```python
from build123d import *

# Parameters (mm, degrees)
F0_R     = 1.5
F1_DEPTH = 11
F2_W     = 61
F2_H     = 1
F2_H_2   = 18
F3_DEPTH = 15
F4_DEPTH = 1
F5_DEPTH = 10.5


with BuildPart() as f1:
    # F0 (on Top) → F1 (new body, symmetric)
    with BuildSketch(Plane.XY):
        Polygon((-4.5, 30.5), (-15, 30.5), (-15, -30.5), (-4.5, -30.5), (4.5, -30.5), (15, -30.5), (15, 30.5), (4.5, 30.5), align=None)
        with Locations((-5.5, -27.5)):
            Circle(F0_R, mode=Mode.SUBTRACT)
        with Locations((5.5, -27.5)):
            Circle(F0_R, mode=Mode.SUBTRACT)
        with Locations((-5.5, 27.5)):
            Circle(F0_R, mode=Mode.SUBTRACT)
        with Locations((5.5, 27.5)):
            Circle(F0_R, mode=Mode.SUBTRACT)
        with Locations((5.5, -27.5)):
            Circle(F0_R)
        with Locations((-5.5, -27.5)):
            Circle(F0_R)
        with Locations((-5.5, 27.5)):
            Circle(F0_R)
        with Locations((5.5, 27.5)):
            Circle(F0_R)
        Polygon((-3.5, 31.5), (-4.5, 30.5), (4.5, 30.5), (3.5, 31.5), align=None)
        Polygon((4.5, -30.5), (-4.5, -30.5), (-3.5, -31.5), (3.5, -31.5), align=None)
    extrude(amount=F1_DEPTH, both=True)

    # F2 (on Right) → F3 (cut, symmetric)
    with BuildSketch(Plane.YZ):
        with Locations((0, 9.5)):
            Rectangle(F2_W, F2_H)
        Rectangle(F2_W, F2_H_2)
        with Locations((0, -9.5)):
            Rectangle(F2_W, F2_H)
    extrude(amount=F3_DEPTH, both=True, mode=Mode.SUBTRACT)

    # F2 (on Right) → F4 (join, symmetric)
    with BuildSketch(Plane.YZ):
        with Locations((0, 9.5)):
            Rectangle(F2_W, F2_H)
        Rectangle(F2_W, F2_H_2)
        with Locations((0, -9.5)):
            Rectangle(F2_W, F2_H)
    extrude(amount=F4_DEPTH, both=True)

    # F0 (on Top) → F5 (cut, symmetric)
    with BuildSketch(Plane.XY):
        with Locations((-5.5, -27.5)):
            Circle(F0_R)
        with Locations((5.5, -27.5)):
            Circle(F0_R)
        with Locations((5.5, 27.5)):
            Circle(F0_R)
        with Locations((-5.5, 27.5)):
            Circle(F0_R)
    extrude(amount=F5_DEPTH, both=True, mode=Mode.SUBTRACT)


solid = f1.part
```
Verification items for the finished model (mm, model axes). A direction names the side the tool comes from. Coordinates: 2 decimals unless noted, no trailing zeros. Order: outer loops, then holes, each group sorted by start corner. A loop starts at its lowest first (then second) coordinate and runs counter-clockwise, first axis right, second up. Notation, with made-up numbers: (14.25, 56) -> (66.25, 56) arc R30 ccw to (66.25, 85) -> close; hole circle Ø9 at (-29.5, 74.25). An arc over 180 degrees is marked (long way). Put each result on its own line as item: value. Start each with the question number.
1) Tool access check on faces 1 (the flat face through (8, 0, -10)), 2 (the flat face through (0, 31.5, 0)), 3 (the flat face through (-1, 0, 0)), 4 (the flat face through (-6, -27, -10.5)). Record the directions out of +Z, -Z, +X, -X, +Y, -Y that give a thin tool (end or side, any length) a straight path to the whole face; none if there is none.
2) Release check for a two-part mould opening along Z. For faces 5 (the flat face through (0, 0, 11)), 6 (the cylindrical face through (5.305, 28.987, 10.246)), 7 (the flat face through (0, 0, -11)), 8 (the flat face through (0, -31.5, 0)) record: pulls with the +Z half, pulls with the -Z half, needs draft (parallel to the pull), parting line crosses it, or undercut.
3) Cross-section at B-B (z = -8.5). Enter the section's corners in (x, y), plus the area to 3 significant figures.
4) Cross-section at D-D (y = 27.5). Enter the section's corners in (x, z).
5) Cross-section at A-A (x = 5.5). Enter the section's corners in (y, z), plus the area to 3 significant figures.
6) Cross-section at C-C (x = 10.25). Enter the section's corners in (y, z), plus the area to 3 significant figures.
7) Material ranges on L1, parallel to Y at x = 5.5, z = 10.15; L2, parallel to X at y = -27.5, z = 10.3; L3, parallel to Y at x = 1.5, z = -2.25, recorded low to high.
8) Go/stop test with flat-tipped pins: pin 1 (6 mm diameter, centred on x = 10, z = -3.5, fed in from +Y); pin 2 (1.1 mm diameter, centred on x = 7.5, z = -10.5, fed in from +Y); pin 3 (10 mm diameter, centred on y = -5, z = -0.5, fed in from +X); pin 4 (10 mm diameter, centred on y = -13, z = -3.5, fed in from -X). Record where each tip stops, or that it passes through.
Geometry check:
1. face 1: +X
1. face 2: +Z, -Z, +X, -X, +Y
1. face 3: -X
1. face 4: none
2. face 5: pulls with the +Z half
2. face 6: undercut
2. face 7: pulls with the -Z half
2. face 8: needs draft
3. outline: (-4.5, -30.5) -> (-3.5, -31.5) -> (3.5, -31.5) -> (4.5, -30.5) -> (1, -30.5) -> (1, 30.5) -> (4.5, 30.5) -> (3.5, 31.5) -> (-3.5, 31.5) -> (-4.5, 30.5) -> (-1, 30.5) -> (-1, -30.5) -> close
3. area: 138 mm^2
4. outline: (-15, -11) -> (15, -11) -> (15, -10) -> (7, -10) -> (7, -10.5) -> (4, -10.5) -> (4, -10) -> (1, -10) -> (1, 10) -> (4, 10) -> (4, 10.5) -> (7, 10.5) -> (7, 10) -> (15, 10) -> (15, 11) -> (-15, 11) -> (-15, 10) -> (-7, 10) -> (-7, 10.5) -> (-4, 10.5) -> (-4, 10) -> (-1, 10) -> (-1, -10) -> (-4, -10) -> (-4, -10.5) -> (-7, -10.5) -> (-7, -10) -> (-15, -10) -> close
5. outline: (-30.5, -11) -> (30.5, -11) -> (30.5, -10) -> (29, -10) -> (29, -10.5) -> (26, -10.5) -> (26, -10) -> (-26, -10) -> (-26, -10.5) -> (-29, -10.5) -> (-29, -10) -> (-30.5, -10) -> close; (-30.5, 10) -> (-29, 10) -> (-29, 10.5) -> (-26, 10.5) -> (-26, 10) -> (26, 10) -> (26, 10.5) -> (29, 10.5) -> (29, 10) -> (30.5, 10) -> (30.5, 11) -> (-30.5, 11) -> close
5. area: 116 mm^2
6. outline: (-30.5, -11) -> (30.5, -11) -> (30.5, -10) -> (-30.5, -10) -> close; (-30.5, 10) -> (30.5, 10) -> (30.5, 11) -> (-30.5, 11) -> close
6. area: 122 mm^2
7. L1: y = -30.5 to -29, -26 to 26, 29 to 30.5
7. L2: x = -15 to -7, -4 to 4, 7 to 15
7. L3: y = -31.5 to -30.5, 30.5 to 31.5
8. pin 1: passes through
8. pin 2: stops at y = 30.5
8. pin 3: stops at x = 1
8. pin 4: stops at x = -1
